```python
from build123d import *

# Parameters (mm, degrees)
BOSS_EXTRUDE1_DEPTH = 1
SKETCH2_R           = 0.95
SKETCH2_R_2         = 0.85
CUT_EXTRUDE1_DEPTH  = 1
SKETCH3_R           = 1.15
CUT_EXTRUDE2_DEPTH  = 1


with BuildPart() as part:
    # Sketch1 → Boss-Extrude1 (new body)
    with BuildSketch(Plane(origin=(0, 0, 0), x_dir=(1, 0, 0), z_dir=(0, 1, 0))):
        Polygon((30, -6.890061842), (5, -6.890061842), (0, -1.890061842), (0, 25.109938158), (8, 33.109938158), (27, 33.109938158), (35, 25.109938158), (35, -1.890061842), align=None)
    extrude(amount=BOSS_EXTRUDE1_DEPTH)

    # Sketch2 → Cut-Extrude1 (cut)
    with BuildSketch(Plane(origin=(0, 1, 0), x_dir=(1, 0, 0), z_dir=(0, 1, 0))):
        with Locations(Location((32.5, -0.890061842, 0), (0, 0, 270))):
            Circle(SKETCH2_R)
        with Locations(Location((2.5, -0.890061842, 0), (0, 0, 270))):
            Circle(SKETCH2_R)
        with Locations(Location((32.5, 24.109938158, 0), (0, 0, 270))):
            Circle(SKETCH2_R)
        with Locations(Location((2.5, 24.109938158, 0), (0, 0, 270))):
            Circle(SKETCH2_R_2)
    extrude(amount=-CUT_EXTRUDE1_DEPTH, mode=Mode.SUBTRACT)

    # Sketch3 → Cut-Extrude2 (cut)
    with BuildSketch(Plane(origin=(0, 1, 0), x_dir=(1, 0, 0), z_dir=(0, 1, 0))):
        with Locations(Location((26, 31.109938158, 0), (0, 0, 270))):
            Circle(SKETCH3_R)
        with Locations(Location((9, 31.109938158, 0), (0, 0, 270))):
            Circle(SKETCH3_R)
    extrude(amount=-CUT_EXTRUDE2_DEPTH, mode=Mode.SUBTRACT)


solid = part.part
```
Verification items for the finished model (mm, model axes). Coordinates: 2 decimals unless noted, no trailing zeros. Loops run counter-clockwise (first coordinate to the right, second up) from the corner with the lowest first, then second, coordinate; pieces in that order, holes last. Notation, with made-up numbers: (50, -18) -> (57, -18) arc R18 ccw to (57, 0) -> close; hole circle Ø2 at (77.25, -29.5). An arc over 180 degrees is marked (long way). Answer in a Markdown table with one row per item. Add a question column.
1. Section check A-A, the plane x = 9. Enter the section's corners in (y, z).
2. Depth check by flat-ended pin: P1, Ø2, axis at x = 26, z = -31.11, coming from the -Y side; P2, Ø1.5, axis at x = 12.5, z = -10, coming from the -Y side. Enter the tip coordinate at first touch or a pass-through.
3. Section check B-B, the plane y = 0.55. Enter the section's corners in (x, z).
4. Section check C-C, the plane x = 2.5. Enter the section's corners in (y, z), then the cut area to 3 significant figures.
5. Section check D-D, the plane x = 25.5. Enter the section's corners in (y, z), then the cut area to 3 significant figures.
6. Draft check along X on faces 1 (the face through (1.98, 0.51, -24.78)), 2 (the face through (18, 0, -13)), 3 (the face through (30.94, 0.49, -29.17)). Enter one of: +X half, -X half, draft (parallel to the pull), parting line (faces both ways), or undercut.
7. Material ranges on probe 1 along Z at (x, y) = (33, 0.3); probe 2 along Z at (x, y) = (3.5, 0.9); probe 3 along Z at (x, y) = (10, 0.6), recorded low to high. Write a range as [from, to].
Derived:
| question | item | result |
|---|---|---|
| 1 | outline | (0, -33.11) -> (1, -33.11) -> (1, -32.26) -> (0, -32.26) -> close; (0, -29.96) -> (1, -29.96) -> (1, 6.89) -> (0, 6.89) -> close |
| 2 | P1 | passes through |
| 2 | P2 | stops at y = 0 |
| 3 | outline | (0, -25.11) -> (8, -33.11) -> (27, -33.11) -> (35, -25.11) -> (35, 1.89) -> (30, 6.89) -> (5, 6.89) -> (0, 1.89) -> close; hole circle Ø1.9 at (2.5, 0.89); hole circle Ø1.7 at (2.5, -24.11); hole circle Ø2.3 at (9, -31.11); hole circle Ø2.3 at (26, -31.11); hole circle Ø1.9 at (32.5, -24.11); hole circle Ø1.9 at (32.5, 0.89) |
| 4 | outline | (0, -27.61) -> (1, -27.61) -> (1, -24.96) -> (0, -24.96) -> close; (0, -23.26) -> (1, -23.26) -> (1, -0.06) -> (0, -0.06) -> close; (0, 1.84) -> (1, 1.84) -> (1, 4.39) -> (0, 4.39) -> close |
| 4 | area | 28.4 mm² |
| 5 | outline | (0, -33.11) -> (1, -33.11) -> (1, -32.15) -> (0, -32.15) -> close; (0, -30.07) -> (1, -30.07) -> (1, 6.89) -> (0, 6.89) -> close |
| 5 | area | 37.9 mm² |
| 6 | face 1 | undercut |
| 6 | face 2 | draft |
| 6 | face 3 | +X half |
| 7 | probe 1 | z = [-27.11, -24.92], [-23.3, 0.08], [1.7, 3.89] |
| 7 | probe 2 | z = [-28.61, 5.39] |
| 7 | probe 3 | z = [-33.11, -31.68], [-30.54, 6.89] |
